Read the model definition and answer for the solid it produces. Units are mm, in the model's axes. Coordinates: 2 decimals unless noted, no trailing zeros. Order: outer loops, then holes, each group sorted by start corner. A loop starts at its lowest first (then second) coordinate and runs counter-clockwise, first axis right, second up.
from build123d import *

# Parameters (mm, degrees)
SKETCH1_W             = 25.4
SKETCH1_H             = 45.295
BOSS_EXTRUDE1_DEPTH   = 3.175
SKETCH2_R             = 4.5
CUT_EXTRUDE1_DEPTH    = 27.158743878
M3X0_5_TAPPED_HOLE1_D = 2.5
FILLET1_R             = 3.175


with BuildPart() as part:
    # Sketch1 → Boss-Extrude1 (new body)
    with BuildSketch(Plane.XY):
        Rectangle(SKETCH1_W, SKETCH1_H)
    extrude(amount=BOSS_EXTRUDE1_DEPTH)

    # Sketch2 → Cut-Extrude1 (cut, through all)
    with BuildSketch(Plane.XY.offset(3.175)):
        with Locations((0, 9.3975)):
            Circle(SKETCH2_R)
    extrude(amount=-CUT_EXTRUDE1_DEPTH, mode=Mode.SUBTRACT)

    # M3x0.5 Tapped Hole1 (through all)
    with Locations(Plane.XY.offset(3.175)):
        with Locations((0, 17.8975), (0, 0.8975)):
            Hole(M3X0_5_TAPPED_HOLE1_D / 2)

    # Fillet1
    fillet1_edges = [part.edges().sort_by_distance(p)[0] for p in [
        (12.7, -22.6475, 1.5875),
        (-12.7, -22.6475, 1.5875),
        (-12.7, 22.6475, 1.5875),
        (12.7, 22.6475, 1.5875),
    ]]
    fillet(fillet1_edges, radius=FILLET1_R)


solid = part.part
Q1. Straight lines are drawn through the part: L1, parallel to Y at x = 0, z = 2.35; L2, parallel to Y at x = -0.75, z = 2; L3, parallel to Y at x = -3, z = 2.55. For each, find the intervals that lie inside material, in ascending order.
Q2. The part is cut by section D-D, the plane z = 2.35. State how many separate pieces and enclosed holes the cut face has, then the cut area to 3 significant figures.
Q3. The part is cut by section B-B, the plane y = 6. Determine the outline of the cut face in (x, z) (3 decimals).
Q4. The part is cut by section A-A, the plane x = 0. Determine the outline of the cut face in (y, z) (1 decimal), then the cut area to 3 significant figures.
Q5. Determine the mould class of faces 1 (the cylindrical face through (-0.59, 13.86, 1.61)), 2 (the flat face through (-12.7, 0, 2)), 3 (the flat face through (0, -22.648, 2)) for opening direction Y: +Y half, -Y half, draft (parallel to the pull), parting line (faces both ways), or undercut.
Q6. The part is cut by section C-C, the plane x = -4. Determine the outline of the cut face in (y, z) (1 decimal), then the cut area to 3 significant figures.
Computed values:
1. L1: y = -22.65 to -0.35, 2.15 to 4.9, 13.9 to 16.65, 19.15 to 22.65
1. L2: y = -22.65 to -0.1, 1.9 to 4.96, 13.83 to 16.9, 18.9 to 22.65
1. L3: y = -22.65 to 6.04, 12.75 to 22.65
2. separate pieces: 1
2. enclosed holes: 3
2. area: 1,070 mm2
3. outline: (-12.7, 0) - (-2.951, 0) - (-2.951, 3.175) - (-12.7, 3.175) - close; (2.951, 0) - (12.7, 0) - (12.7, 3.175) - (2.951, 3.175) - close
4. outline: (-22.6, 0) - (-0.4, 0) - (-0.4, 3.2) - (-22.6, 3.2) - close; (2.1, 0) - (4.9, 0) - (4.9, 3.2) - (2.1, 3.2) - close; (13.9, 0) - (16.6, 0) - (16.6, 3.2) - (13.9, 3.2) - close; (19.1, 0) - (22.6, 0) - (22.6, 3.2) - (19.1, 3.2) - close
4. area: 99.4 mm2
5. face 1: undercut
5. face 2: draft
5. face 3: -Y half
6. outline: (-22.6, 0) - (7.3, 0) - (7.3, 3.2) - (-22.6, 3.2) - close; (11.5, 0) - (22.6, 0) - (22.6, 3.2) - (11.5, 3.2) - close
6. area: 131 mm2
